Verification items for the finished model (mm, model axes). Give positions to 0.01 mm unless a question says otherwise; leave off trailing zeros. Order: outer loops, then holes, each group sorted by start corner. A loop starts at its lowest first (then second) coordinate and runs counter-clockwise, first axis right, second up. Notation, with made-up numbers: (18.25, -32.75) - (48.25, -32.75) arc R10 ccw to (48.25, -27.75) - close; hole circle Ø4 at (31, 30). An arc over 180 degrees is marked (long way). Answer as a JSON object with one key per item and string values.
```python
from build123d import *

# Parameters (mm, degrees)
F0_W     = 79.4
F0_H     = 24
F1_DEPTH = 4
F2_R     = 5.5
F3_DEPTH = 25
F4_R     = 3


with BuildPart() as f1:
    # F0 (on Front) → F1 (new body)
    with BuildSketch(Plane.XZ):
        Rectangle(F0_W, F0_H)
    extrude(amount=F1_DEPTH)

    # F2 (on face) → F3 (cut)
    with BuildSketch(Plane.XZ.offset(4)):
        with Locations((-27.2, 0)):
            Circle(F2_R)
        with Locations((27.2, 0)):
            Circle(F2_R)
    extrude(amount=-F3_DEPTH, mode=Mode.SUBTRACT)

    # F4
    f4_edges = [f1.edges().sort_by_distance(p)[0] for p in [
        (39.7, -2, 12),
        (39.7, -2, -12),
        (-39.7, -2, -12),
        (-39.7, -2, 12),
    ]]
    fillet(f4_edges, radius=F4_R)


solid = f1.part
```
(1) Section check C-C (y = -1.75). Record the cut outline in (x, z), then the cut area to 3 significant figures.
Computed values:
{"outline": "(-39.7, -9) arc R3 ccw to (-36.7, -12) - (36.7, -12) arc R3 ccw to (39.7, -9) - (39.7, 9) arc R3 ccw to (36.7, 12) - (-36.7, 12) arc R3 ccw to (-39.7, 9) - close; hole circle Ø11 at (-27.2, 0); hole circle Ø11 at (27.2, 0)", "area": "1,710 mm²"}
(2) Gauge pin test, flat end, axial feed: pin 1 Ø9 at (x, z) = (27.2, 0) entering from -Y. Record the tip position at first contact, or that the pin passes through.
Computed values:
{"pin 1": "passes through"}
(3) Section check A-A (x = -27.2). Record the cut outline in (y, z), then the cut area to 3 significant figures.
Computed values:
{"outline": "(-4, -12) - (0, -12) - (0, -5.5) - (-4, -5.5) - close; (-4, 5.5) - (0, 5.5) - (0, 12) - (-4, 12) - close", "area": "52.0 mm²"}
(4) Release check for a two-part mould opening along X. For faces 1 (the cylindrical face through (-38.84, -2.03, -11.1)), 2 (the flat face through (-1, -2, -12)), 3 (the cylindrical face through (38.8, -2.03, -11.14)), 4 (the cylindrical face through (-22.12, -2.03, -2.11)) record: pulls with the +X half, pulls with the -X half, needs draft (parallel to the pull), parting line crosses it, or undercut.
Computed values:
{"face 1": "pulls with the -X half", "face 2": "needs draft", "face 3": "pulls with the +X half", "face 4": "undercut"}
(5) Material ranges on line 1 along Z through (x, y) = (-27.2, -1.2); line 2 along X through (y, z) = (-2, -3); line 3 along X through (y, z) = (-3.65, 2.75), recorded low to high. Write a range as [from, to].
Computed values:
{"line 1": "z = [-12, -5.5], [5.5, 12]", "line 2": "x = [-39.7, -31.81], [-22.59, 22.59], [31.81, 39.7]", "line 3": "x = [-39.7, -31.96], [-22.44, 22.44], [31.96, 39.7]"}
(6) Section check B-B (z = 0). Record the cut outline in (x, y).
Computed values:
{"outline": "(-39.7, -4) - (-32.7, -4) - (-32.7, 0) - (-39.7, 0) - close; (-21.7, -4) - (21.7, -4) - (21.7, 0) - (-21.7, 0) - close; (32.7, -4) - (39.7, -4) - (39.7, 0) - (32.7, 0) - close"}
